Solid Edge part; units mm, degrees
sketch "Sketch1" plane through (0, 0, 0) normal (1, 0, 0) x (0, 1, 0)
  line L0 (-38.0473, 37.2787) -> (-38.0473, 25.4787)
  line L1 (-38.0473, 25.4787) -> (110.9527, 25.4787)
  line L2 (110.9527, 25.4787) -> (110.9527, 37.2787)
  line L3 (110.9527, 37.2787) -> (-38.0473, 37.2787)
  dimension "D1" = 110.9527
  dimension "D2" = 38.0473
extrude "Protrusion1" add sketch "Sketch1" against normal blind 1
hole "Hole_1" at (0, -15.0473, 31.3787) direction (-1, 0, 0) diameter 4.5 end through all
hole "Hole1" at (0, 89.9527, 31.3787) direction (-1, 0, 0) diameter 4.5 end through all
hole "Hole2" at (0, -27.0473, 31.3787) direction (-1, 0, 0) diameter 4.5 end through all
The model under review builds one solid part; all positions refer to its coordinate system, in mm. Give positions to 0.01 mm unless a question says otherwise; leave off trailing zeros. Write each loop counter-clockwise with the first axis right and the second up, starting at its lowest first coordinate (ties: lowest second). Pieces come first, ordered by that corner, then holes. Notation, with made-up numbers: (49, 31) -> (71, 31) arc R29 cw to (71, 52) -> close; hole circle Ø1 at (45, -25). An arc over 180 degrees is marked (long way). Put each result on its own line as item: value.
(1) For pin 1 Ø2 at (y, z) = (52, 31) entering from +X, flat-tipped, find the tip position at first contact; note if it passes through.
Results are:
pin 1: x = 0
(2) We need section A-A, the plane z = 31.25. Give the boundary of the cut face in (x, y), and give its area (3 significant figures).
Results are:
outline: (-1, -38.05) -> (0, -38.05) -> (0, -29.29) -> (-1, -29.29) -> close; (-1, -24.8) -> (0, -24.8) -> (0, -17.29) -> (-1, -17.29) -> close; (-1, -12.8) -> (0, -12.8) -> (0, 87.71) -> (-1, 87.71) -> close; (-1, 92.2) -> (0, 92.2) -> (0, 110.95) -> (-1, 110.95) -> close
area: 136 mm²
(3) The part is to be moulded in two halves that separate along Y. For faces 1 (the cylindrical face through (-0.493, -17.043, 30.34)), 2 (the flat face through (0, 35, 31)), say which applies: pulls with the +Y half, pulls with the -Y half, needs draft (parallel to the pull), parting line crosses it, or undercut.
Results are:
face 1: undercut
face 2: needs draft
(4) To check wall thickness, follow probe 1 along Y at (x, z) = (-0.8, 31.5); probe 2 along Y at (x, z) = (-0.6, 32); probe 3 along Z at (x, y) = (-0.1, -26). State the ranges of each line that lie inside material, in increasing order. Write a range as from..to.
Results are:
probe 1: -38.05..-29.29, -24.8..-17.29, -12.8..87.71, 92.2..110.95
probe 2: -38.05..-29.21, -24.88..-17.21, -12.88..87.79, 92.12..110.95
probe 3: 25.48..29.39, 33.37..37.28
(5) We need section B-B, the plane x = -0.3. Give the boundary of the cut face in (y, z), and give its area (3 significant figures).
Results are:
outline: (-38.05, 25.48) -> (110.95, 25.48) -> (110.95, 37.28) -> (-38.05, 37.28) -> close; hole circle Ø4.5 at (-27.05, 31.38); hole circle Ø4.5 at (-15.05, 31.38); hole circle Ø4.5 at (89.95, 31.38)
area: 1,710 mm²
